Print and shaded views of the part. All mm, measured from the part's lowest x, y and z. A direction names the side the tool comes from. Coordinates: 2 decimals unless noted, no trailing zeros. Loops run counter-clockwise (first coordinate to the right, second up) from the corner with the lowest first, then second, coordinate; pieces in that order, holes last. Notation, with made-up numbers: M -26,87 L -8,87 A12 cw -8,107 Z; hole C 87.25,85 d3. An arc over 180 degrees is marked long. Answer as CSV lines item,"result". Start each with the question number.
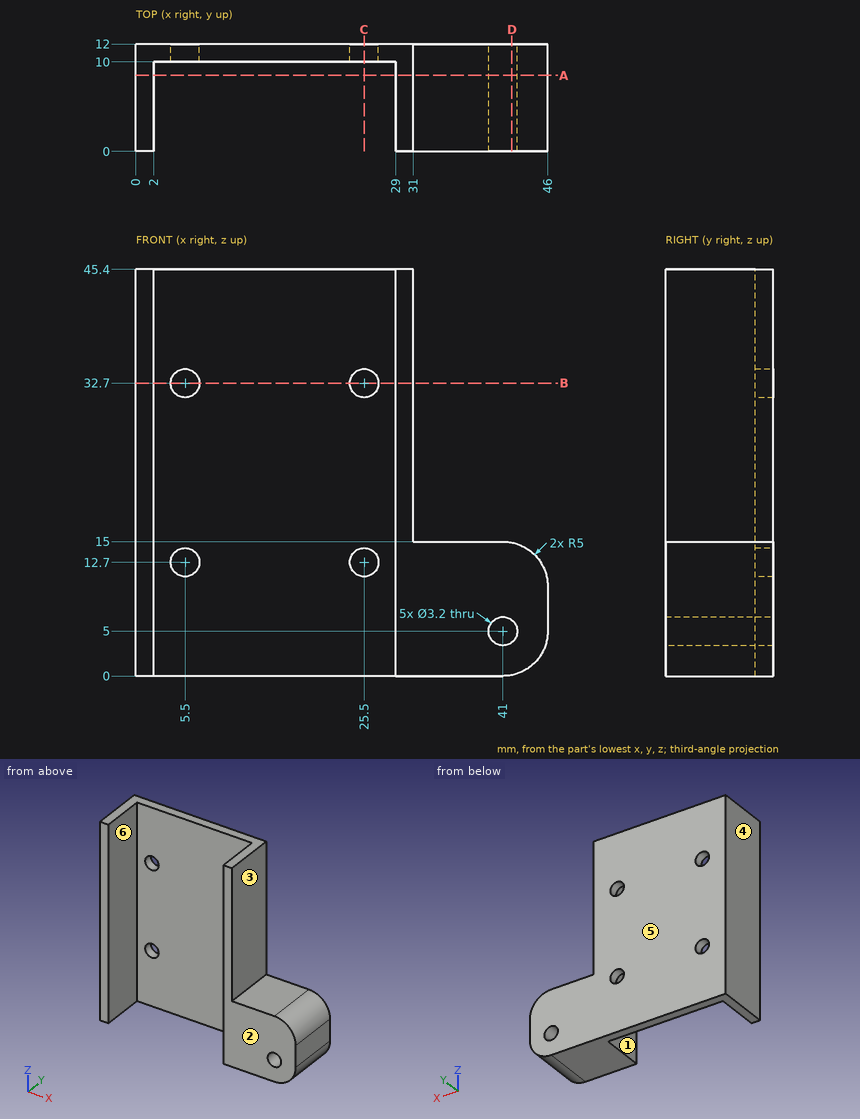
Q1. Flat gauge pins, fed straight in: P1, Ø3, axis at x = 17, y = 10.5, coming from the -Z side; P2, Ø4, axis at x = 5.5, z = 32.7, coming from the -Y side; P3, Ø3.5, axis at y = 6.5, z = 35.5, coming from the +X side. Where does each tip first touch, or does it go through?
Q2. Slice it at D-D, the plane x = 42. Write the cut outline in (y, z), and give its area (3 significant figures).
Q3. Slice it at C-C, the plane x = 25.5. Write the cut outline in (y, z), and give its area (3 significant figures).
Q4. Slice it at B-B, the plane z = 32.7. Write the cut outline in (x, y).
Q5. Tool access for the marked faces 1, 2 and 3: list every direction of +Z, -Z, +X, -X, +Y, -Y with a clear straight run to the whole face (end or side of a thin tool).
Q6. Two-plate mould, pull along X, no slides. Class the marked faces 4, 5 and 6: +X half, -X half, draft (parallel to the pull), parting line (faces both ways), or undercut.
Q7. Slice it at A-A, the plane y = 8.5. Write the cut outline in (x, z).
Q8. Wall check: L1, parallel to X at y = 11.2, z = 32.7; L2, parallel to X at y = 5.25, z = 5; L3, parallel to Z at x = 5.5, y = 11.4. Give the ranges that are in metal, low to high.
Solved:
1,P1,"stops at z = 0"
1,P2,"stops at y = 10"
1,P3,"stops at x = 31"
2,outline,"M 0,0.1 L 12,0.1 L 12,3.75 L 0,3.75 Z; M 0,6.25 L 12,6.25 L 12,14.9 L 0,14.9 Z"
2,area,"148 mm2"
3,outline,"M 10,0 L 12,0 L 12,11.1 L 10,11.1 Z; M 10,14.3 L 12,14.3 L 12,31.1 L 10,31.1 Z; M 10,34.3 L 12,34.3 L 12,45.4 L 10,45.4 Z"
3,area,"78.0 mm2"
4,outline,"M 0,0 L 2,0 L 2,10 L 3.9,10 L 3.9,12 L 0,12 Z; M 7.1,10 L 23.9,10 L 23.9,12 L 7.1,12 Z; M 27.1,10 L 29,10 L 29,0 L 31,0 L 31,12 L 27.1,12 Z"
5,face 1,"+Z, -Z, -Y"
5,face 2,"+Z, -Z, +X, -X, -Y"
5,face 3,"+Z, +X, +Y, -Y"
6,face 4,"-X half"
6,face 5,"draft"
6,face 6,"undercut"
7,outline,"M 0,0 L 2,0 L 2,45.4 L 0,45.4 Z; M 29,0 L 41,0 A5 ccw 46,5 L 46,10 A5 ccw 41,15 L 31,15 L 31,45.4 L 29,45.4 Z; hole C 41,5 d3.2"
8,L1,"x = 0 to 3.9, 7.1 to 23.9, 27.1 to 31"
8,L2,"x = 0 to 2, 29 to 39.4, 42.6 to 46"
8,L3,"z = 0 to 11.1, 14.3 to 31.1, 34.3 to 45.4"
